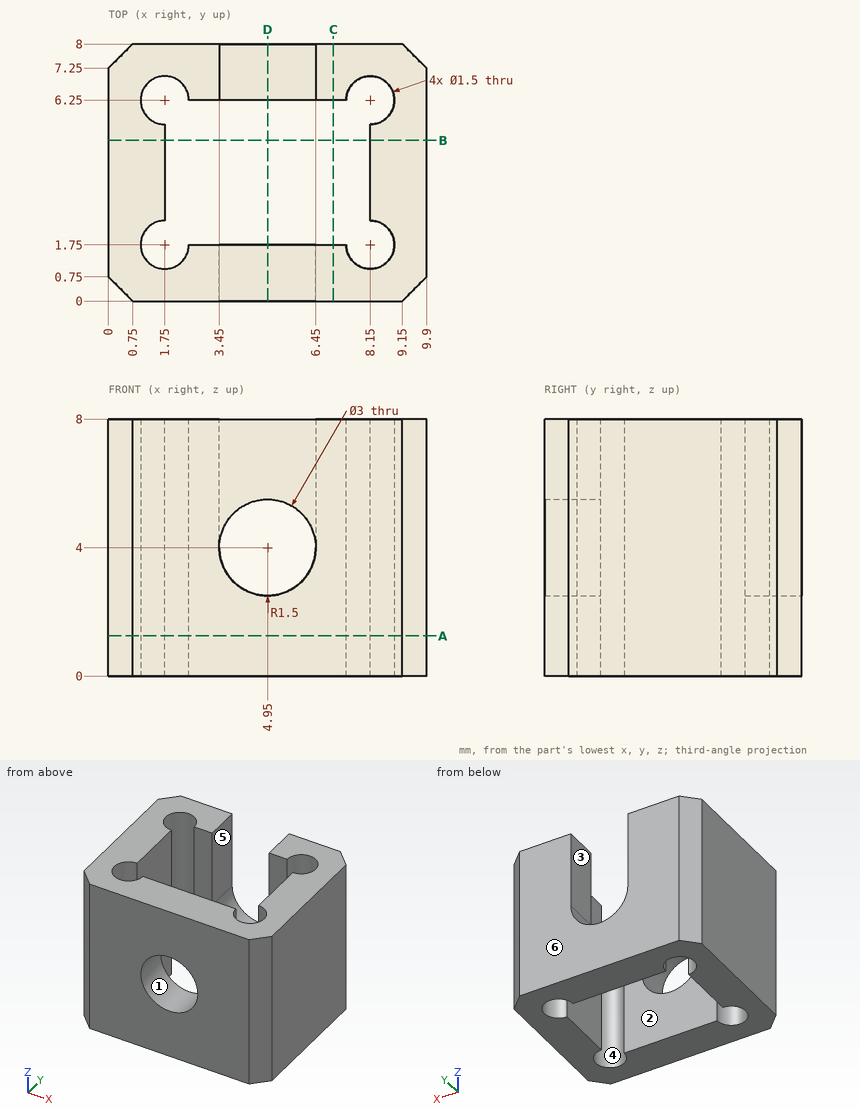
Verification items for this drawing (mm, ordinates from the low corner). A direction names the side the tool comes from. Coordinates: 2 decimals unless noted, no trailing zeros. Order: outer loops, then holes, each group sorted by start corner. A loop starts at its lowest first (then second) coordinate and runs counter-clockwise, first axis right, second up. Notation, with made-up numbers: (47, -13.5) - (81, -13.5) arc R26 ccw to (81, 16.5) - close; hole circle Ø8 at (81.25, 33). An arc over 180 degrees is marked (long way). Answer in a Markdown table with one row per item. Add a question column.
1. Section check C-C (x = 7). Enter the section's corners in (y, z).
2. Material ranges on L1, parallel to Y at x = 3, z = 1.75; L2, parallel to X at y = 4.5, z = 7.5; L3, parallel to X at y = 0.85, z = 4, recorded low to high. Write a range as [from, to].
3. Section check D-D (x = 4.95). Enter the section's corners in (y, z).
4. Section check B-B (y = 5). Enter the section's corners in (x, z).
5. Section check A-A (z = 1.25). Enter the section's corners in (x, y), plus the area to 3 significant figures.
6. Draft check along Y on the marked faces 4, 5 and 6. Enter one of: +Y half, -Y half, draft (parallel to the pull), parting line (faces both ways), or undercut.
7. Access from +Z, -Z, +X, -X, +Y, -Y to the whole of each face (thin tool, end or side, straight path). Record for the marked faces 1, 2 and 3.
Data:
| question | item | result |
|---|---|---|
| 1 | outline | (0, 0) - (1.75, 0) - (1.75, 8) - (0, 8) - close; (6.25, 0) - (8, 0) - (8, 8) - (6.25, 8) - close |
| 2 | L1 | y = [0, 1.75], [6.25, 8] |
| 2 | L2 | x = [0, 1.75], [8.15, 9.9] |
| 2 | L3 | x = [0, 3.45], [6.45, 9.9] |
| 3 | outline | (0, 0) - (1.75, 0) - (1.75, 2.5) - (0, 2.5) - close; (0, 5.5) - (1.75, 5.5) - (1.75, 8) - (0, 8) - close; (6.25, 0) - (8, 0) - (8, 2.5) - (6.25, 2.5) - close |
| 4 | outline | (0, 0) - (1.75, 0) - (1.75, 8) - (0, 8) - close; (8.15, 0) - (9.9, 0) - (9.9, 8) - (8.15, 8) - close |
| 5 | outline | (0, 0.75) - (0.75, 0) - (9.15, 0) - (9.9, 0.75) - (9.9, 7.25) - (9.15, 8) - (0.75, 8) - (0, 7.25) - close; hole (1.75, 2.5) arc R0.75 ccw (long way) to (2.5, 1.75) - (7.4, 1.75) arc R0.75 ccw (long way) to (8.15, 2.5) - (8.15, 5.5) arc R0.75 ccw (long way) to (7.4, 6.25) - (2.5, 6.25) arc R0.75 ccw (long way) to (1.75, 5.5) - close |
| 5 | area | 44.0 mm² |
| 6 | face 4 | undercut |
| 6 | face 5 | draft |
| 6 | face 6 | +Y half |
| 7 | face 1 | +Y, -Y |
| 7 | face 2 | +Z, -Z |
| 7 | face 3 | +Z, +Y |
